from build123d import *

# Parameters (mm, degrees)
F1_DEPTH = 6.35
F2_R     = 1.5875
F3_DEPTH = 1.525


with BuildPart() as f1:
    # F0 (on Front) → F1 (new body)
    with BuildSketch(Plane.XZ):
        with BuildLine():
            Line((-13.335, 0), (-6.604, 0))
            ThreePointArc((-6.604, 0), (-6.559286, 0.767195), (-6.425748, 1.524))
            Line((-6.425748, 1.524), (-9.251668, 1.524))
            Line((-9.251668, 1.524), (-13.335, 1.524))
            Line((-13.335, 1.524), (-13.335, 0))
        make_face()
        with BuildLine():
            Line((-6.604, 0), (-5.08, 0))
            ThreePointArc((-5.08, 0), (-3.592102, 3.592102), (0, 5.08))
            ThreePointArc((0, 5.08), (3.592102, 3.592102), (5.08, 0))
            Line((5.08, 0), (6.604, 0))
            ThreePointArc((6.604, 0), (6.559286, 0.767195), (6.425748, 1.524))
            ThreePointArc((6.425748, 1.524), (4.095627, 5.180604), (0, 6.604))
            ThreePointArc((0, 6.604), (-4.095627, 5.180604), (-6.425748, 1.524))
            ThreePointArc((-6.425748, 1.524), (-6.559286, 0.767195), (-6.604, 0))
        make_face()
        with BuildLine():
            ThreePointArc((6.425748, 1.524), (6.559286, 0.767195), (6.604, 0))
            Line((6.604, 0), (13.335, 0))
            Line((13.335, 0), (13.335, 1.524))
            Line((13.335, 1.524), (9.251668, 1.524))
            Line((9.251668, 1.524), (6.425748, 1.524))
        make_face()
    extrude(amount=F1_DEPTH)

    # F2 (on face) → F3 (cut, through all)
    with BuildSketch(Plane.XY.offset(1.524)):
        with Locations((10.16, -3.175)):
            Circle(F2_R)
        with Locations((-10.16, -3.175)):
            Circle(F2_R)
    extrude(amount=-F3_DEPTH, mode=Mode.SUBTRACT)


solid = f1.part
Can you work these out from the model? Positions are in its coordinate system, mm. A direction names the side the tool comes from. Coordinates: 2 decimals unless noted, no trailing zeros. Loops run counter-clockwise (first coordinate to the right, second up) from the corner with the lowest first, then second, coordinate; pieces in that order, holes last. Notation, with made-up numbers: (88, 88.5) - (137, 88.5) arc R30 ccw to (137, 117.5) - close; hole circle Ø3 at (42, 66.25). An arc over 180 degrees is marked (long way). Answer as a JSON object with one key per item and string values. Group by question number.
Item 1: For pin 1 (1.5 mm diameter, centred on y = -2.5, z = 4, fed in from +X); pin 2 (3 mm diameter, centred on x = 1.5, y = -2.5, fed in from +Z); pin 3 (2 mm diameter, centred on y = -3, z = 4, fed in from -X); pin 4 (1 mm diameter, centred on y = -4.5, z = 5.5, fed in from +X), each with a flat end and sliding along its axis, tell me the tip position at first contact or that it passes through.
Item 2: If we section it at D-D (y = -1): List the corners of the cut face in (x, z) for me (3 decimals), plus the area to 3 significant figures.
Item 3: If I drill on L1, parallel to X at y = -4.25, z = 0.5 (3 decimals); L2, parallel to X at y = -2, z = 0.5 (3 decimals); L3, parallel to Y at x = 10.16, z = 0.6, over which ranges is the centre line in solid material (lowest first)? Write a range as from..to.
Item 4: If we mould it in two halves opening along X, with no side actions, what happens to faces 4 (the face through (-1.1, -6.35, 5.3)), 5 (the face through (8.574, -3.105, 0.773)), 6 (the face through (-13.335, -3, 1))? For each: released by +X, released by -X, zero draft, split by the parting line, or undercut.
Item 5: If we section it at B-B (x = -10.16): List the corners of the cut face in (y, z) for me.
Item 6: On a 3-axis mill with a long thin cutter (end or side, diameter ignored), from which of +Z, -Z, +X, -X, +Y, -Y can I reach the whole of each face in a straight line? I mean faces 1 (the face through (8, -3, 1.524)), 2 (the face through (-1.1, 0, 5.3)), 3 (the face through (-8, -3, 1.524)). Say none if no direction works.
Item 7: If we section it at C-C (y = -2): List the corners of the cut face in (x, z) for me (3 decimals).
Item 8: If we section it at A-A (z = 0.5): State how many separate pieces and enclosed holes the cut face has, plus the area to 3 significant figures.
Returned:
{
 "1": {"pin 1": "stops at x = 5.75", "pin 2": "stops at z = 6.6", "pin 3": "stops at x = -5.88", "pin 4": "stops at x = 4.31"},
 "2": {"outline": "(-13.335, 0) - (-5.08, 0) arc R5.08 cw to (0, 5.08) arc R5.08 cw to (5.08, 0) - (13.335, 0) - (13.335, 1.524) - (6.426, 1.524) arc R6.604 ccw to (0, 6.604) arc R6.604 ccw to (-6.426, 1.524) - (-13.335, 1.524) - close", "area": "48.7 mm²"},
 "3": {"L1": "x = -13.335..-11.328, -8.992..-5.055, 5.055..8.992, 11.328..13.335", "L2": "x = -13.335..-11.227, -9.093..-5.055, 5.055..9.093, 11.227..13.335", "L3": "y = -6.35..-4.76, -1.59..0"},
 "4": {"face 4": "zero draft", "face 5": "undercut", "face 6": "released by -X"},
 "5": {"outline": "(-6.35, 0) - (-4.76, 0) - (-4.76, 1.52) - (-6.35, 1.52) - close; (-1.59, 0) - (0, 0) - (0, 1.52) - (-1.59, 1.52) - close"},
 "6": {"face 1": "+Z, +X, +Y, -Y", "face 2": "+Z, -Z, +X, -X, +Y", "face 3": "+Z, -X, +Y, -Y"},
 "7": {"outline": "(-13.335, 0) - (-11.227, 0) - (-11.227, 1.524) - (-13.335, 1.524) - close; (-9.093, 0) - (-5.08, 0) arc R5.08 cw to (0, 5.08) arc R5.08 cw to (5.08, 0) - (9.093, 0) - (9.093, 1.524) - (6.426, 1.524) arc R6.604 ccw to (0, 6.604) arc R6.604 ccw to (-6.426, 1.524) - (-9.093, 1.524) - close; (11.227, 0) - (13.335, 0) - (13.335, 1.524) - (11.227, 1.524) - close"},
 "8": {"separate pieces": "2", "enclosed holes": "2", "area": "89.3 mm²"}
}
